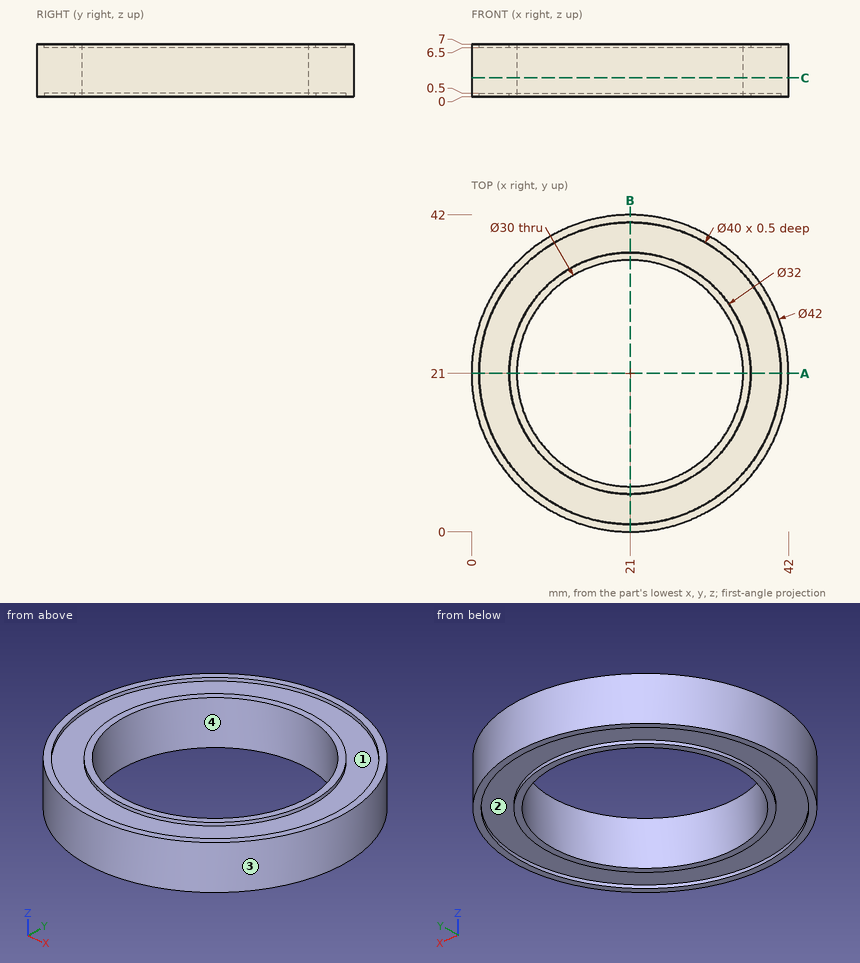
Geometry: see drawing. Coordinates: mm, zero at the bounding-box minimum. A direction names the side the tool comes from. Round coordinates to 2 decimals unless told otherwise and drop trailing zeros. Loops run counter-clockwise (first coordinate to the right, second up) from the corner with the lowest first, then second, coordinate; pieces in that order, holes last. Notation, with made-up numbers: M 48,19.25 L 56,19.25 A20 cw 56,27.25 Z; hole C 67,29.5 d6. An arc over 180 degrees is marked long. Use a Markdown table: item, result. Add a question column.
1. Cut plane A-A, the plane y = 21. Output: boundary loops of the cut face in (x, z), and give its area (3 significant figures).
2. Ray query, line 1 along Y through (x, z) = (21, 0.35); line 2 along Y through (x, z) = (21, 1.5); line 3 along Z through (x, y) = (22.5, 39.5). Return the intervals inside material, ascending. Write a range as [from, to].
3. Pull-direction query (Y, two-part tool) for the marked faces 3 and 4; classes: +Y half, -Y half, draft (parallel to the pull), parting line (faces both ways), or undercut.
4. Set-up query: the marked faces 1 and 2. Return all of +Z, -Z, +X, -X, +Y, -Y with unobstructed straight access to the full face (end or side cutting, diameter ignored); none if empty.
5. Cut plane C-C, the plane z = 2.5. Output: boundary loops of the cut face in (x, y).
6. Contact query for a flat-ended pin moving along its axis: pin 1 (4 mm diameter, centred on x = 28, z = 4.5, fed in from -Y). Output: stop coordinate, or through.
Solution:
| question | item | result |
|---|---|---|
| 1 | outline | M 0,0 L 1,0 L 1,0.5 L 5,0.5 L 5,0 L 6,0 L 6,7 L 5,7 L 5,6.5 L 1,6.5 L 1,7 L 0,7 Z; M 36,0 L 37,0 L 37,0.5 L 41,0.5 L 41,0 L 42,0 L 42,7 L 41,7 L 41,6.5 L 37,6.5 L 37,7 L 36,7 Z |
| 1 | area | 76.0 mm2 |
| 2 | line 1 | y = [0, 1], [5, 6], [36, 37], [41, 42] |
| 2 | line 2 | y = [0, 6], [36, 42] |
| 2 | line 3 | z = [0.5, 6.5] |
| 3 | face 3 | parting line |
| 3 | face 4 | undercut |
| 4 | face 1 | +Z |
| 4 | face 2 | -Z |
| 5 | outline | C 21,21 d42; hole C 21,21 d30 |
| 6 | pin 1 | stops at y = 0.6 |
